Can you work these out from the drawing? Everything is in mm from the part's minimum corner. A direction names the side the tool comes from. Give positions to 0.01 mm unless a question says otherwise; leave off trailing zeros. Loops run counter-clockwise (first coordinate to the right, second up) from the corner with the lowest first, then second, coordinate; pieces in that order, holes last. Notation, with made-up numbers: (52, 25.5) -> (106, 25.5) arc R17 cw to (106, 58.5) -> close; hole circle Ø1 at (76, 80.5). An arc over 180 degrees is marked (long way). Return JSON: item names as keys, results as strings. Group by question number.
Q1. I need wall thicknesses on line 1 along X through (y, z) = (5, 10); line 2 along Z through (x, y) = (10, 10); line 3 along X through (y, z) = (6, 13.75). Which ranges of each line are inside material? Lowest first, please. Write a range as [from, to].
Q2. Suppose I cut it at D-D, the plane z = 4. Please give me the cut outline in (x, y), and give its area (3 significant figures).
Q3. Thinking about a two-plate mould opening in Z: for the marked faces 1, 2 and 3, which applies, pulls with the +Z half, pulls with the -Z half, needs draft (parallel to the pull), parting line crosses it, or undercut?
Q4. Suppose I cut it at B-B, the plane x = 10. Please give me the cut outline in (y, z).
Q5. Suppose I cut it at C-C, the plane z = 10. Please give me the cut outline in (x, y), and give its area (4 significant figures).
Q6. Suppose I cut it at A-A, the plane y = 3. Please give me the cut outline in (x, z), and give its area (3 significant figures).
Q7. Will these pins go through, and if not, where does the flat tip stop? pin 1 (2 mm diameter, centred on x = 32, y = 6, fed in from -Z); pin 2 (4 mm diameter, centred on y = 9, z = 15, fed in from +X).
Q8. Which directions (+Z, -Z, +X, -X, +Y, -Y) give clear straight access to the entire face, cutting with the end or side of a thin tool? Please do the marked faces 4 and 5.
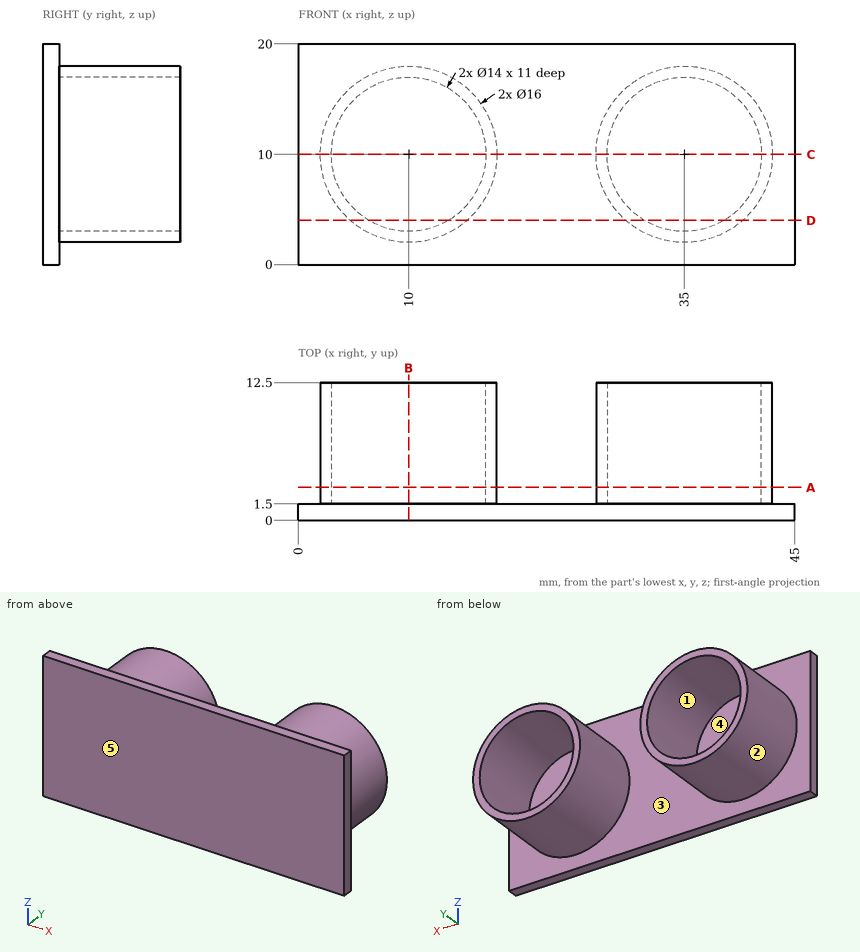
Ans:
{
 "1": {"line 1": "x = [2, 3], [17, 18], [27, 28], [42, 43]", "line 2": "z = [2, 3], [17, 18]", "line 3": "x = [2.93, 4.09], [15.91, 17.07], [27.93, 29.09], [40.91, 42.07]"},
 "2": {"outline": "(0, 0) -> (45, 0) -> (45, 1.5) -> (40.29, 1.5) -> (40.29, 12.5) -> (38.61, 12.5) -> (38.61, 1.5) -> (31.39, 1.5) -> (31.39, 12.5) -> (29.71, 12.5) -> (29.71, 1.5) -> (15.29, 1.5) -> (15.29, 12.5) -> (13.61, 12.5) -> (13.61, 1.5) -> (6.39, 1.5) -> (6.39, 12.5) -> (4.71, 12.5) -> (4.71, 1.5) -> (0, 1.5) -> close", "area": "142 mm^2"},
 "3": {"face 1": "undercut", "face 2": "parting line crosses it", "face 3": "needs draft"},
 "4": {"outline": "(0, 0) -> (1.5, 0) -> (1.5, 2) -> (12.5, 2) -> (12.5, 3) -> (1.5, 3) -> (1.5, 17) -> (12.5, 17) -> (12.5, 18) -> (1.5, 18) -> (1.5, 20) -> (0, 20) -> close"},
 "5": {"outline": "(0, 0) -> (45, 0) -> (45, 1.5) -> (43, 1.5) -> (43, 12.5) -> (42, 12.5) -> (42, 1.5) -> (28, 1.5) -> (28, 12.5) -> (27, 12.5) -> (27, 1.5) -> (18, 1.5) -> (18, 12.5) -> (17, 12.5) -> (17, 1.5) -> (3, 1.5) -> (3, 12.5) -> (2, 12.5) -> (2, 1.5) -> (0, 1.5) -> close", "area": "111.5 mm^2"},
 "6": {"outline": "circle Ø16 at (10, 10); circle Ø16 at (35, 10); hole circle Ø14 at (10, 10); hole circle Ø14 at (35, 10)", "area": "94.2 mm^2"},
 "7": {"pin 1": "stops at z = 2.25", "pin 2": "stops at x = 42.42"},
 "8": {"face 4": "+Y", "face 5": "+Z, -Z, +X, -X, -Y"}
}
